Design review of the part built by this model. Coordinates are the model's own, in mm. A direction names the side the tool comes from. Coordinates: 2 decimals unless noted, no trailing zeros. Loops run counter-clockwise (first coordinate to the right, second up) from the corner with the lowest first, then second, coordinate; pieces in that order, holes last. Notation, with made-up numbers: (45, 14.5) - (71, 14.5) arc R17 ccw to (71, 20.5) - close; hole circle Ø3 at (23.5, 34). An arc over 180 degrees is marked (long way). One line per question, with ' | ' between items.
from build123d import *

# Parameters (mm, degrees)
SKETCH1_W                 = 94.7166
SKETCH1_H                 = 56.007
EXTRUDE1_DEPTH            = 24.765
SKETCH2_W                 = 58.0644
SKETCH2_H                 = 43.4594
EXTRUDE2_DEPTH            = 0.127
SKETCH3_W                 = 6.858
SKETCH3_H                 = 5.588
EXTRUDE3_DEPTH            = 0.381
LPATTERN1_COUNT           = 3
LPATTERN1_PITCH           = 8.89
LPATTERN2_COUNT           = 3
LPATTERN2_PITCH           = 12.7
LPATTERN2_COPY_1_SKETCH_W = 6.858
LPATTERN2_COPY_1_SKETCH_H = 5.588
LPATTERN2_COPY_1_DEPTH    = 0.381
LPATTERN2_COPY_2_SKETCH_W = 6.858
LPATTERN2_COPY_2_SKETCH_H = 5.588
LPATTERN2_COPY_2_DEPTH    = 0.381
LPATTERN2_COPY_3_SKETCH_W = 6.858
LPATTERN2_COPY_3_SKETCH_H = 5.588
LPATTERN2_COPY_3_DEPTH    = 0.381
LPATTERN2_COPY_4_SKETCH_W = 6.858
LPATTERN2_COPY_4_SKETCH_H = 5.588
LPATTERN2_COPY_4_DEPTH    = 0.381
SKETCH4_R                 = 1.524
SKETCH4_R_2               = 2.54
SKETCH4_W                 = 4.953
SKETCH4_H                 = 16.51
SKETCH4_W_2               = 7.62
SKETCH4_H_2               = 21.59
EXTRUDE4_DEPTH            = 0.381
SKETCH5_R                 = 2.286
SKETCH5_W                 = 15.24
SKETCH5_H                 = 4.572
SKETCH5_W_2               = 12.7
SKETCH5_W_3               = 25.4
SKETCH5_H_2               = 6.604
EXTRUDE5_DEPTH            = 0.381
SKETCH6_W                 = 2.794
SKETCH6_H                 = 25.2984
EXTRUDE6_DEPTH            = 28.321


with BuildPart() as part:
    # Sketch1 → Extrude1 (new body)
    with BuildSketch(Plane.XY):
        Rectangle(SKETCH1_W, SKETCH1_H)
    extrude(amount=EXTRUDE1_DEPTH)

    # Sketch2 → Extrude2 (add)
    with BuildSketch(Plane.XY.offset(24.765)):
        with Locations((11.9761, 1.1938)):
            Rectangle(SKETCH2_W, SKETCH2_H)
        with BuildLine():
            Line((-38.950442947, 26.0985), (-32.600442947, 26.0985))
            ThreePointArc((-32.600442947, 26.0985), (-29.425442947, 22.9235), (-32.600442947, 19.7485))
            Line((-32.600442947, 19.7485), (-38.950442947, 19.7485))
            ThreePointArc((-38.950442947, 19.7485), (-42.125442947, 22.9235), (-38.950442947, 26.0985))
        make_face()
    extrude(amount=EXTRUDE2_DEPTH)

    # Sketch3 → Extrude3 (add)
    with BuildSketch(Plane.XY.offset(24.765)):
        with Locations((-24.2951, 12.5095)):
            Rectangle(SKETCH3_W, SKETCH3_H)
    extrude3 = extrude(amount=EXTRUDE3_DEPTH)

    # LPattern1: Extrude3 ×3
    with Locations(*[(-i * LPATTERN1_PITCH, 0, 0) for i in range(1, LPATTERN1_COUNT)]):
        add(extrude3)

    # LPattern2: Extrude3 ×3
    with Locations(*[(0, -i * LPATTERN2_PITCH, 0) for i in range(1, LPATTERN2_COUNT)]):
        add(extrude3)

    # LPattern2 copy 1 sketch → LPattern2 copy 1 (add)
    with BuildSketch(Plane(origin=(-8.89, -12.7, 24.765), x_dir=(1, 0, 0), z_dir=(0, 0, 1))):
        with Locations((-24.2951, 12.5095)):
            Rectangle(LPATTERN2_COPY_1_SKETCH_W, LPATTERN2_COPY_1_SKETCH_H)
    extrude(amount=LPATTERN2_COPY_1_DEPTH)

    # LPattern2 copy 2 sketch → LPattern2 copy 2 (add)
    with BuildSketch(Plane(origin=(-8.89, -25.4, 24.765), x_dir=(1, 0, 0), z_dir=(0, 0, 1))):
        with Locations((-24.2951, 12.5095)):
            Rectangle(LPATTERN2_COPY_2_SKETCH_W, LPATTERN2_COPY_2_SKETCH_H)
    extrude(amount=LPATTERN2_COPY_2_DEPTH)

    # LPattern2 copy 3 sketch → LPattern2 copy 3 (add)
    with BuildSketch(Plane(origin=(-17.78, -12.7, 24.765), x_dir=(1, 0, 0), z_dir=(0, 0, 1))):
        with Locations((-24.2951, 12.5095)):
            Rectangle(LPATTERN2_COPY_3_SKETCH_W, LPATTERN2_COPY_3_SKETCH_H)
    extrude(amount=LPATTERN2_COPY_3_DEPTH)

    # LPattern2 copy 4 sketch → LPattern2 copy 4 (add)
    with BuildSketch(Plane(origin=(-17.78, -25.4, 24.765), x_dir=(1, 0, 0), z_dir=(0, 0, 1))):
        with Locations((-24.2951, 12.5095)):
            Rectangle(LPATTERN2_COPY_4_SKETCH_W, LPATTERN2_COPY_4_SKETCH_H)
    extrude(amount=LPATTERN2_COPY_4_DEPTH)

    # Sketch4 → Extrude4 (add)
    with BuildSketch(Plane.ZY.offset(47.3583)):
        with Locations(Location((12.192, -6.4135, 0), (0, 0, 180))):
            Circle(SKETCH4_R)
        with Locations(Location((12.192, -16.3195, 0), (0, 0, 180))):
            Circle(SKETCH4_R_2)
        with Locations((21.427500813, 9.5885)):
            Rectangle(SKETCH4_W, SKETCH4_H)
        with Locations((10.922, 10.9855)):
            Rectangle(SKETCH4_W_2, SKETCH4_H_2)
    extrude(amount=EXTRUDE4_DEPTH)

    # Sketch5 → Extrude5 (add)
    with BuildSketch(Plane.XZ.offset(28.0035)):
        with Locations(Location((-9.2583, 14.351, 0), (0, 0, 90))):
            Circle(SKETCH5_R)
        with Locations((-24.4983, 14.097)):
            Rectangle(SKETCH5_W, SKETCH5_H)
        with Locations((4.7117, 14.097)):
            Rectangle(SKETCH5_W_2, SKETCH5_H)
        with Locations((25.5397, 13.081)):
            Rectangle(SKETCH5_W_3, SKETCH5_H_2)
    extrude(amount=EXTRUDE5_DEPTH)

    # Sketch6 → Extrude6 (cut)
    with BuildSketch(Plane(origin=(47.3583, 0, 0), x_dir=(0, 0, -1), z_dir=(1, 0, 0))):
        with Locations((-18.796, -4.1783)):
            Rectangle(SKETCH6_W, SKETCH6_H)
    extrude(amount=-EXTRUDE6_DEPTH, mode=Mode.SUBTRACT)


solid = part.part
Q1. Draft analysis for pull direction Y (two halves, no side actions). For faces 6 (the flat face through (-24, 13, 25.146)), 7 (the flat face through (5, -28.384, 14)), 8 (the flat face through (33, -4, 20.193)), state which applies: +Y half, -Y half, draft (parallel to the pull), parting line (faces both ways), or undercut.
Returned:
face 6: draft | face 7: -Y half | face 8: undercut
Q2. To check wall thickness, follow line 1 along Z through (x, y) = (20, 3); line 2 along Z through (x, y) = (43.5, 6) (3 decimals); line 3 along Y through (x, z) = (-2, 3.5). State the ranges of each line that lie inside material, in increasing order.
Returned:
line 1: z = 0 to 17.4, 20.19 to 24.89 | line 2: z = 0 to 17.399, 20.193 to 24.765 | line 3: y = -28 to 28
Q3. Take a section at C-C (y = 4.5). Give the boundary of the cut face in (x, z) (3 decimals), plus the area to 3 significant figures.
Returned:
outline: (-47.739, 7.112) - (-47.358, 7.112) - (-47.358, 0) - (47.358, 0) - (47.358, 17.399) - (19.037, 17.399) - (19.037, 20.193) - (47.358, 20.193) - (47.358, 24.765) - (41.008, 24.765) - (41.008, 24.892) - (-17.056, 24.892) - (-17.056, 24.765) - (-47.358, 24.765) - (-47.358, 23.904) - (-47.739, 23.904) - (-47.739, 18.951) - (-47.358, 18.951) - (-47.358, 14.732) - (-47.739, 14.732) - close | area: 2,280 mm²
Q4. Tool access review of faces 1 (the flat face through (-36, 23, 24.892)), 2 (the flat face through (33, 8.471, 19)), 3 (the cylindrical face through (-9.945, -28.191, 16.531)), 4 (the flat face through (12, 1, 24.892)), 5 (the cylindrical face through (-47.55, -18.84, 12.52)): name each direction out of +Z, -Z, +X, -X, +Y, -Y from which nothing blocks a thin tool from reaching the whole face with its end or side.
Returned:
face 1: +Z, +X, -X, +Y | face 2: +X | face 3: -Y | face 4: +Z, +X, +Y, -Y | face 5: -X
Q5. For pin 1 (17 mm diameter, centred on x = 10, y = 3, fed in from +Z); pin 2 (2 mm diameter, centred on y = -0.5, z = 15.5, fed in from -X), all flat-tipped, find the tip position at first contact; note any pin that passes through.
Returned:
pin 1: stops at z = 24.89 | pin 2: stops at x = -47.36
